Input: part model. Units: mm. Frame: model coordinates. Face numbers are marked on the shaded views. Round coordinates to 2 decimals unless told otherwise and drop trailing zeros. Order: outer loops, then holes, each group sorted by start corner. A loop starts at its lowest first (then second) coordinate and runs counter-clockwise, first axis right, second up. Notation, with made-up numbers: M 88.5,-25 L 95.5,-25 A33 ccw 95.5,5 Z; hole C -6,-17.5 d5. An arc over 180 degrees is marked long. One line per question, with ' | ' between items.
```python
from build123d import *

# Parameters (mm, degrees)
ESQUISSE1_W             = 28
ESQUISSE1_H             = 4
BOSS_EXTRU_1_DEPTH      = 20
ESQUISSE2_R             = 1.2
ENL_V_MAT_EXTRU_1_DEPTH = 35.641016151
ESQUISSE3_R             = 3
ESQUISSE3_R_2           = 1.173644897
ENL_V_MAT_EXTRU_3_DEPTH = 35.641016151
ESQUISSE4_W             = 4
ESQUISSE4_H             = 4
ENL_V_MAT_EXTRU_4_DEPTH = 2


with BuildPart() as part:
    # Esquisse1 → Boss.-Extru.1 (new body)
    with BuildSketch(Plane.XY):
        with Locations((14, 2)):
            Rectangle(ESQUISSE1_W, ESQUISSE1_H)
    extrude(amount=BOSS_EXTRU_1_DEPTH)

    # Esquisse2 → Enlèv. mat.-Extru.1 (cut, through all)
    with BuildSketch(Plane.XY.offset(20)):
        with Locations((2, 2)):
            Circle(ESQUISSE2_R)
        with Locations((26, 2)):
            Circle(ESQUISSE2_R)
    extrude(amount=-ENL_V_MAT_EXTRU_1_DEPTH, mode=Mode.SUBTRACT)

    # Esquisse3 → Enlèv. mat.-Extru.3 (cut, through all)
    with BuildSketch(Plane(origin=(0, 4, 0), x_dir=(1, 0, 0), z_dir=(0, 1, 0))):
        with Locations(Location((14, -10, 0), (0, 0, 270))):
            Circle(ESQUISSE3_R)
        with Locations(Location((8.35754662, -6.773125373, 0), (0, 0, 270))):
            Circle(ESQUISSE3_R_2)
        with Locations(Location((19.615782092, -6.726929347, 0), (0, 0, 270))):
            Circle(ESQUISSE3_R_2)
        with Locations(Location((14.026671288, -16.49994528, 0), (0, 0, 270))):
            Circle(ESQUISSE3_R_2)
    extrude(amount=-ENL_V_MAT_EXTRU_3_DEPTH, mode=Mode.SUBTRACT)

    # Esquisse4 → Enlèv. mat.-Extru.4 (cut)
    with BuildSketch(Plane.XY.offset(20)):
        with Locations((2, 2)):
            Rectangle(ESQUISSE4_W, ESQUISSE4_H)
        with Locations((26, 2)):
            Rectangle(ESQUISSE4_W, ESQUISSE4_H)
    extrude(amount=-ENL_V_MAT_EXTRU_4_DEPTH, mode=Mode.SUBTRACT)


solid = part.part
```
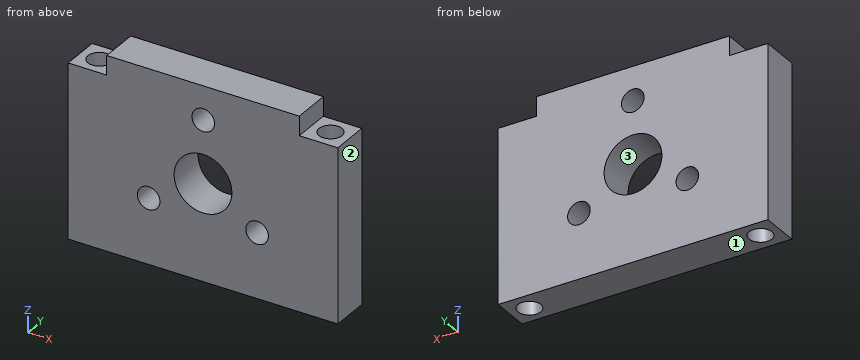
Item 1: First-contact query: pin 1 (4 mm diameter, centred on x = 14.03, z = 16.5, fed in from +Y); pin 2 (1.9 mm diameter, centred on x = 8.36, z = 6.77, fed in from -Y); pin 3 (1.2 mm diameter, centred on x = 25.5, y = 2.5, fed in from +Z); pin 4 (1.6 mm diameter, centred on y = 2, z = 19, fed in from +X). Flat tips, straight axial feed; report the tip coordinate or a pass-through.
Report:
pin 1: y = 4 | pin 2: through | pin 3: z = 18 | pin 4: x = 24
Item 2: Section query B-B, the plane y = 1.55. Return loops of the section in (x, z), plus the area to 3 significant figures.
Report:
outline: M 0,0 L 0.89,0 L 0.89,18 L 0,18 Z; M 3.11,0 L 24.89,0 L 24.89,18 L 24,18 L 24,20 L 4,20 L 4,18 L 3.11,18 Z; M 27.11,0 L 28,0 L 28,18 L 27.11,18 Z; hole C 8.36,6.77 d2.35; hole C 14,10 d6; hole C 14.03,16.5 d2.35; hole C 19.62,6.73 d2.35 | area: 423 mm²
Item 3: Section query A-A, the plane z = 10. Return loops of the section in (x, y), plus the area to 3 significant figures.
Report:
outline: M 0,0 L 11,0 L 11,4 L 0,4 Z; M 17,0 L 28,0 L 28,4 L 17,4 Z; hole C 2,2 d2.4; hole C 26,2 d2.4 | area: 79.0 mm²
Item 4: Line query: line 1 along X through (y, z) = (1.9, 5.5); line 2 along Y through (x, z) = (26, 11.25); line 3 along X through (y, z) = (2.8, 7.75). Output: solid intervals per line, ascending. Write a range as from..to.
Report:
line 1: 0..0.8, 3.2..24.8, 27.2..28 | line 2: 0..0.8, 3.2..4 | line 3: 0..1.11, 2.89..7.71, 9.01..12.02, 15.98..19.04, 20.19..25.11, 26.89..28
Item 5: Mould query, pull axis Z, two halves, no side actions, for the marked faces 1, 2 and 3. Classes: +Z half, -Z half, draft (parallel to the pull), parting line (faces both ways), or undercut.
Report:
face 1: -Z half | face 2: draft | face 3: undercut
Item 6: Section query C-C, the plane x = 26. Return loops of the section in (y, z), plus the area to 3 significant figures.
Report:
outline: M 0,0 L 0.8,0 L 0.8,18 L 0,18 Z; M 3.2,0 L 4,0 L 4,18 L 3.2,18 Z | area: 28.8 mm²
Item 7: Section query D-D, the plane z = 14. Return loops of the section in (x, y).
Report:
outline: M 0,0 L 28,0 L 28,4 L 0,4 Z; hole C 2,2 d2.4; hole C 26,2 d2.4
